```python
from build123d import *

# Parameters (mm, degrees)
ESQUISSE1_W                  = 12.75
ESQUISSE1_H                  = 5.77
BASE_EXTRUSION_DEPTH         = 5.95
ENL_V_MAT_EXTRU_1_DEPTH      = 1.68
COQUE1_OUTLINE_W             = 10.15
COQUE1_OUTLINE_H             = 4.77
COQUE1_DEPTH                 = 5.45
COQUE1_2_OUTLINE_W           = 1.6
COQUE1_2_OUTLINE_H           = 4.77
COQUE1_2_DEPTH               = 3.77
ENL_V_MAT_EXTRU_2_DEPTH      = 10.185115677
ENL_V_MAT_EXTRU_3_DEPTH      = 10.185115677
ENL_V_MAT_EXTRU_3_DEPTH_BACK = 10.185115677
ESQUISSE4_W                  = 2
ESQUISSE4_H                  = 0.5
ESQUISSE4_W_2                = 0.5
ESQUISSE4_H_2                = 1
ESQUISSE5_W                  = 1.2
ESQUISSE5_H                  = 3
ENL_V_MAT_EXTRU_4_DEPTH      = 10.185115677


# Read off the part's stored shape, not the designer's step: Coque1
with BuildPart() as part:
    # Esquisse1 → Base-Extrusion (new body)
    with BuildSketch(Plane.XY):
        Rectangle(ESQUISSE1_W, ESQUISSE1_H)
    extrude(amount=BASE_EXTRUSION_DEPTH)

    # Esquisse2 → Enlèv. mat.-Extru.1 (cut)
    with BuildSketch(Plane.XY.offset(5.95)):
        Polygon((-5.675, 2), (-4.775, 2), (-4.775, -2), (-5.675, -2), (-5.675, -1.18), (-6.375, -1.18), (-6.375, 1.18), (-5.675, 1.18), align=None)
    extrude(amount=-ENL_V_MAT_EXTRU_1_DEPTH, mode=Mode.SUBTRACT)

    # Coque1 outline → Coque1 (cut)
    with BuildSketch(Plane.XY):
        with Locations((0.8, 0)):
            Rectangle(COQUE1_OUTLINE_W, COQUE1_OUTLINE_H)
    extrude(amount=COQUE1_DEPTH, mode=Mode.SUBTRACT)

    # Coque1 2 outline → Coque1 2 (cut)
    with BuildSketch(Plane.XY):
        with Locations((-5.075, 0)):
            Rectangle(COQUE1_2_OUTLINE_W, COQUE1_2_OUTLINE_H)
    extrude(amount=COQUE1_2_DEPTH, mode=Mode.SUBTRACT)

    # Esquisse3 → Enlèv. mat.-Extru.2 (cut, symmetric)
    with BuildSketch(Plane(origin=(0, 0, 0), x_dir=(1, 0, 0), z_dir=(0, 1, 0))):
        with BuildLine():
            Line((6.375, -2), (3, -2))
            ThreePointArc((3, -2), (2.116116524, -1.633883476), (1.75, -0.75))
            Line((1.75, -0.75), (1.75, 0))
            Line((1.75, 0), (6.375, 0))
            Line((6.375, 0), (6.375, -2))
        make_face()
    enl_v_mat_extru_2 = extrude(amount=ENL_V_MAT_EXTRU_2_DEPTH, both=True, mode=Mode.SUBTRACT)

    # Symétrie1: Enlèv. mat.-Extru.2 across plane
    add(enl_v_mat_extru_2.mirror(Plane(origin=(0, 0, 0), x_dir=(0, 0, 1), z_dir=(1, 0, 0))), mode=Mode.SUBTRACT)

    # Esquisse4 → Enlèv. mat.-Extru.3 (cut, two sides: drawn at the far end of the back side and taken through both)
    with BuildSketch(Plane(origin=(0, 0, 0), x_dir=(1, 0, 0), z_dir=(0, 1, 0)).offset(-ENL_V_MAT_EXTRU_3_DEPTH_BACK)):
        with Locations((0, -1)):
            Rectangle(ESQUISSE4_W, ESQUISSE4_H)
        with Locations((-5.225, -5)):
            Rectangle(ESQUISSE4_W_2, ESQUISSE4_H_2)
    extrude(amount=ENL_V_MAT_EXTRU_3_DEPTH + ENL_V_MAT_EXTRU_3_DEPTH_BACK, mode=Mode.SUBTRACT)

    # Esquisse5 → Enlèv. mat.-Extru.4 (cut, through all)
    with BuildSketch(Plane.XY.offset(5.95)):
        with Locations((-1.875, 0)):
            Rectangle(ESQUISSE5_W, ESQUISSE5_H)
    extrude(amount=-ENL_V_MAT_EXTRU_4_DEPTH, mode=Mode.SUBTRACT)


solid = part.part
```
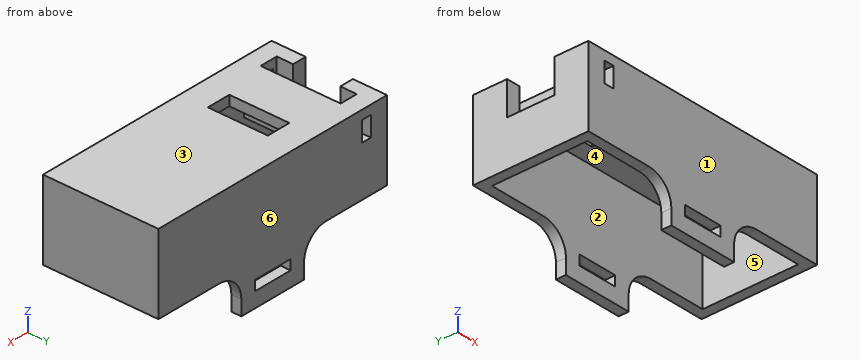
For this review, take the finished solid that the model builds, in its own axes (mm). Face numbers are marked on the shaded views. A direction names the side the tool comes from. Give positions to 0.01 mm unless a question says otherwise; leave off trailing zeros. Order: outer loops, then holes, each group sorted by start corner. A loop starts at its lowest first (then second) coordinate and runs counter-clockwise, first axis right, second up.
1) Wall thickness on line 1 (Y direction, x = -2, z = 3.1) (3 decimals); line 2 (X direction, y = 2.2, z = 2.55) (3 decimals); line 3 (X direction, y = -2.15, z = 5.3) (3 decimals): over which ranges is each line inside the solid? List them lowest first.
2) Insertion check: pin 1 (0.6 mm diameter, centred on y = 2.5, z = 0.5, fed in from +X); pin 2 (1.3 mm diameter, centred on y = 0, z = 5, fed in from -X) (3 decimals). Each pin has a flat end and moves straight along its axis. Give the tip position at first contact, or say it passes through.
3) Take a section at A-A (z = 5). Give the boundary of the cut face in (x, y) (3 decimals), then the cut area to 3 significant figures.
4) Take a section at D-D (y = 2.55). Give the boundary of the cut face in (x, z) (3 decimals).
5) The part is to be moulded in two halves that separate along Y. For the marked faces 3, 4, 5 and 6, say which applies: released by +Y, released by -Y, zero draft, split by the parting line, or undercut.
6) For the marked faces 1 and 2, list the 3-axis set-ups (+Z, -Z, +X, -X, +Y, -Y) from which the entire face can be reached by the end or side of a thin tool; tool diameter is ignored.
7) Take a section at C-C (x = -5.25). Give the boundary of the cut face in (y, z) (3 decimals), then the cut area to 3 significant figures.
8) Take a section at B-B (y = -0.65). Give the boundary of the cut face in (x, z) (3 decimals), then the cut area to 4 significant figures.
Derived:
1. line 1: y = -2.885 to -2.385, 2.385 to 2.885
1. line 2: x = -6.375 to -5.875, 5.875 to 6.375
1. line 3: x = -6.375 to -5.475, -4.975 to -4.275, 5.875 to 6.375
2. pin 1: stops at x = 1.75
2. pin 2: stops at x = -4.775
3. outline: (-6.375, -2.885) - (-5.475, -2.885) - (-5.475, -2) - (-5.675, -2) - (-5.675, -1.18) - (-6.375, -1.18) - close; (-6.375, 1.18) - (-5.675, 1.18) - (-5.675, 2) - (-5.475, 2) - (-5.475, 2.885) - (-6.375, 2.885) - close; (-4.975, -2.885) - (6.375, -2.885) - (6.375, 2.885) - (-4.975, 2.885) - (-4.975, 2) - (-4.775, 2) - (-4.775, -2) - (-4.975, -2) - close; hole (-4.275, -2.385) - (5.875, -2.385) - (5.875, 2.385) - (-4.275, 2.385) - close
3. area: 19.0 mm2
4. outline: (-6.375, 2) - (-3, 2) arc R1.25 cw to (-1.75, 0.75) - (-1.75, 0) - (1.75, 0) - (1.75, 0.75) arc R1.25 cw to (3, 2) - (6.375, 2) - (6.375, 5.95) - (-6.375, 5.95) - close; hole (-5.475, 4.5) - (-4.975, 4.5) - (-4.975, 5.5) - (-5.475, 5.5) - close; hole (-1, 0.75) - (1, 0.75) - (1, 1.25) - (-1, 1.25) - close
5. face 3: zero draft
5. face 4: undercut
5. face 5: undercut
5. face 6: released by +Y
6. face 1: +Z, -Z, +X, -X, -Y
6. face 2: -Z
7. outline: (-2.885, 2) - (-2.385, 2) - (-2.385, 3.77) - (2.385, 3.77) - (2.385, 2) - (2.885, 2) - (2.885, 4.5) - (2, 4.5) - (2, 4.27) - (-2, 4.27) - (-2, 4.5) - (-2.885, 4.5) - close; (-2.885, 5.5) - (-2, 5.5) - (-2, 5.95) - (-2.885, 5.95) - close; (2, 5.5) - (2.885, 5.5) - (2.885, 5.95) - (2, 5.95) - close
7. area: 5.86 mm2
8. outline: (-6.375, 2) - (-5.875, 2) - (-5.875, 3.77) - (-4.275, 3.77) - (-4.275, 5.45) - (-2.475, 5.45) - (-2.475, 5.95) - (-4.775, 5.95) - (-4.775, 4.27) - (-6.375, 4.27) - close; (-1.275, 5.45) - (5.875, 5.45) - (5.875, 2) - (6.375, 2) - (6.375, 5.95) - (-1.275, 5.95) - close
8. area: 9.225 mm2
